Can you work these out from the model? Positions are in its coordinate system, mm. A direction names the side the tool comes from. Round coordinates to 2 decimals unless told otherwise and drop trailing zeros. Write each loop counter-clockwise with the first axis right and the second up, starting at its lowest first coordinate (ties: lowest second). Pieces come first, ordered by that corner, then holes. Notation, with made-up numbers: (21.25, -26.5) -> (64.25, -26.5) arc R27 cw to (64.25, 3.5) -> close; hole circle Ø5 at (1, 4.5). An arc over 180 degrees is marked (long way). Use CSV: the item, a comma, the result in double quotes.
```python
from build123d import *

# Parameters (mm, degrees)
F0_R           = 9
F1_DEPTH       = 15
F1_DEPTH_BACK  = 15
F2_SIZE        = 4
F4_D           = 3
F4_DEPTH       = 10
F4_CSINK_D     = 6
F4_CSINK_ANGLE = 90
F5_R           = 2.5
F6_DEPTH       = 10


with BuildPart() as f1:
    # F0 (on Front) → F1 (new body, two sides)
    with BuildSketch(Plane.XZ) as f1_sk:
        Polygon((0, 10), (0, 0), (50, 0), (50, 10), (40, 10), (40, 92), (10, 92), (10, 10), align=None)
        with Locations((25, 55)):
            Circle(F0_R, mode=Mode.SUBTRACT)
        with Locations((25, 77)):
            Circle(F0_R, mode=Mode.SUBTRACT)
    extrude(amount=F1_DEPTH)
    extrude(f1_sk.sketch, amount=-F1_DEPTH_BACK)

    # F2
    f2_edges = [f1.edges().sort_by_distance(p)[0] for p in [
        (40, 0, 92),
        (10, 0, 92),
    ]]
    chamfer(f2_edges, length=F2_SIZE)

    # F4
    with Locations(Plane.XY.offset(92)):
        with Locations((25, 0)):
            CounterSinkHole(F4_D / 2, F4_CSINK_D / 2, depth=F4_DEPTH, counter_sink_angle=F4_CSINK_ANGLE)

    # F5 (on face) → F6 (cut)
    with BuildSketch(Plane.XY.offset(10)):
        with Locations((5, 10)):
            Circle(F5_R)
        with Locations((5, -10)):
            Circle(F5_R)
        with Locations((45, -10)):
            Circle(F5_R)
        with Locations((45, 10)):
            Circle(F5_R)
    extrude(amount=-F6_DEPTH, mode=Mode.SUBTRACT)


solid = f1.part
```
Q1. On a 3-axis mill with a long thin cutter (end or side, diameter ignored), from which of +Z, -Z, +X, -X, +Y, -Y can I reach the whole of each face in a straight line? I mean faces 5 (the face through (45, 0, 10)), 6 (the face through (5, 0, 10)), 7 (the face through (26.5, 0.07, 88.15)). Say none if no direction works.
Resolved:
face 5,"+Z, +X, +Y, -Y"
face 6,"+Z, -X, +Y, -Y"
face 7,"+Z"
Q2. Suppose I cut it at C-C (z = 77). Write out the boundary of the cut face in (x, y).
Resolved:
outline,"(10, -15) -> (16, -15) -> (16, 15) -> (10, 15) -> close; (34, -15) -> (40, -15) -> (40, 15) -> (34, 15) -> close"
Q3. Will these pins go through, and if not, where does the flat tip stop? P1, Ø5, axis at x = 38, y = -2, coming from the +Z side; P2, Ø4, axis at y = -7.5, z = 62.5, coming from the +X side; P3, Ø3, axis at x = 3, y = 1.5, coming from the +Z side; P4, Ø3, axis at y = 6.5, z = 57.5, coming from the -X side.
Resolved:
P1,"stops at z = 92"
P2,"stops at x = 40"
P3,"stops at z = 10"
P4,"stops at x = 10"
Q4. If we mould it in two halves opening along Y, with no side actions, what happens to faces 1 (the face through (40, 0, 48)), 2 (the face through (25, -15, 36)), 3 (the face through (25, 15, 36)), 4 (the face through (27, 0, 91))? For each: released by +Y, released by -Y, zero draft, split by the parting line, or undercut.
Resolved:
face 1,"zero draft"
face 2,"released by -Y"
face 3,"released by +Y"
face 4,"undercut"
Q5. Suppose I cut it at A-A (x = 45). Write out the boundary of the cut face in (y, z).
Resolved:
outline,"(-15, 0) -> (-12.5, 0) -> (-12.5, 10) -> (-15, 10) -> close; (-7.5, 0) -> (7.5, 0) -> (7.5, 10) -> (-7.5, 10) -> close; (12.5, 0) -> (15, 0) -> (15, 10) -> (12.5, 10) -> close"
Q6. Suppose I cut it at D-D (x = 25). Write out the boundary of the cut face in (y, z).
Resolved:
outline,"(-15, 0) -> (15, 0) -> (15, 46) -> (-15, 46) -> close; (-15, 64) -> (15, 64) -> (15, 68) -> (-15, 68) -> close; (-15, 86) -> (-1.5, 86) -> (-1.5, 90.5) -> (-3, 92) -> (-15, 92) -> close; (1.5, 86) -> (15, 86) -> (15, 92) -> (3, 92) -> (1.5, 90.5) -> close"
Q7. Suppose I cut it at B-B (y = -10). Write out the boundary of the cut face in (x, z).
Resolved:
outline,"(0, 0) -> (2.5, 0) -> (2.5, 10) -> (0, 10) -> close; (7.5, 0) -> (42.5, 0) -> (42.5, 10) -> (40, 10) -> (40, 88) -> (36, 92) -> (14, 92) -> (10, 88) -> (10, 10) -> (7.5, 10) -> close; (47.5, 0) -> (50, 0) -> (50, 10) -> (47.5, 10) -> close; hole circle Ø18 at (25, 55); hole circle Ø18 at (25, 77)"
Q8. Please list where these lines run through material, in increasing order: probe 1 along Z at (x, y) = (25, 8.5); probe 2 along Z at (x, y) = (23, 11); probe 3 along X at (y, z) = (-6, 77).
Resolved:
probe 1,"z = 0 to 46, 64 to 68, 86 to 92"
probe 2,"z = 0 to 46.23, 63.77 to 68.23, 85.77 to 92"
probe 3,"x = 10 to 16, 34 to 40"
